CAD build for the part. Positions are in the model's coordinates, mm. A direction names the side the tool comes from. Coordinates: 2 decimals unless noted, no trailing zeros. Order: outer loops, then holes, each group sorted by start corner. A loop starts at its lowest first (then second) coordinate and runs counter-clockwise, first axis right, second up. Notation, with made-up numbers: (61, -10) -> (89, -10) arc R11 cw to (89, -4) -> close; hole circle Ø9 at (26, 69.25). An arc over 180 degrees is marked (long way). Use one line per item in the form item = value. Start each with the question number.
Autodesk Inventor part; units mm, degrees
ref_plane "YZ Plane" through (0, 0, 0) normal (1, 0, 0) x (0, 1, 0)
ref_plane "XZ Plane" through (0, 0, 0) normal (0, 1, 0) x (-1, 0, 0)
ref_plane "XY Plane" through (0, 0, 0) normal (0, 0, 1) x (1, 0, 0)
sketch "Sketch1" plane through (0, 0, 0) normal (0, 1, 0) x (-1, 0, 0)
  line L0 (15.875, -28.575) -> (-15.875, -28.575)
  line L1 (-15.875, -28.575) -> (-15.875, 28.575)
  line L2 (-15.875, 28.575) -> (15.875, 28.575)
  line L3 (15.875, 28.575) -> (15.875, -28.575)
  line L4 (15.875, -28.575) -> (-15.875, 28.575) construction
  line L5 (-15.875, -28.575) -> (15.875, 28.575) construction
  point P0 (0, 0)
  dimension "d0" = 31.75
  dimension "d1" = 57.15
extrude "Extrusion1" add sketch "Sketch1" along normal blind 9.525
sketch "Sketch2" plane through (0, 9.525, 0) normal (0, 1, 0) x (1, 0, 0)
  line L0 (15.875, -28.575) -> (15.875, 28.575)
  line L1 (-15.875, -28.575) -> (15.875, -28.575)
  line L2 (15.875, 28.575) -> (9.525, 28.575)
  line L3 (9.525, 28.575) -> (9.525, -28.575)
  line L4 (9.525, -28.575) -> (15.875, -28.575)
  line L5 (15.875, -28.575) -> (15.875, 28.575)
  point P0 (0, 0)
  dimension "d4" = 6.35
extrude "Extrusion2" add sketch "Sketch2" along normal blind 12.7
sketch "Sketch3" plane through (0, 0, 0) normal (0, -1, 0) x (1, 0, 0)
  line L0 (-15.875, 28.575) -> (9.525, 28.575)
  point P0 (0, 0)
  point P1 (4.699, -3.175)
  dimension "d14" = 4.826
  dimension "d15" = 31.75
hole "Hole1" at (4.699, 0, -3.175) direction (0, 1, 0) diameter 4.2 end through all counterbore diameter 7.62 counterbore depth 5.08
sketch "Sketch5" plane through (0, 9.525, 0) normal (0, 1, 0) x (1, 0, 0)
  line L0 (9.525, 28.575) -> (-15.875, 28.575)
  circle A0 centre (4.699, 3.175) radius 3.81
  line L1 (-15.875, -28.575) -> (9.525, -28.575)
  point P0 (0, 0)
  point P1 (-8.001, 3.175)
  dimension "d33" = 12.7
  dimension "d40" = 31.75
hole "Hole3" at (-8.001, 9.525, -3.175) direction (0, -1, 0) diameter 4.699 end through all counterbore diameter 7.62 counterbore depth 4.445
sketch "Sketch6" plane through (0, 0, 0) normal (0, -1, 0) x (1, 0, 0)
  circle A0 centre (-8.001, -8.179) radius 1.0125
  circle A1 centre (-8.001, 1.829) radius 1.0125
  circle A2 centre (-8.001, -3.175) radius 2.3495
  point P0 (0, 0)
  dimension "d34" = 2.025
  dimension "d35" = 2.025
  dimension "d36" = 5.004
  dimension "d37" = 5.004
extrude "Extrusion3" cut sketch "Sketch6" against normal blind 4.826 contours A0 | A1
properties part number "Mount for Slit VA100CP"
1) Cut at B-B on z = -4. Give the cut face in (x, y) (3 decimals).
2) Cut at C-C on z = -19. Give the cut face in (x, y) (3 decimals), then the cut area to 3 significant figures.
3) Cut at A-A on y = 3.75. Give the cut face in (x, z) (1 decimal).
4) Drop flat-ended pins along their axis: P1, Ø4, axis at x = -8.001, z = -3.175, coming from the +Y side; P2, Ø3, axis at x = 6, z = -1, coming from the +Y side (3 decimals); P3, Ø5.5, axis at x = 4.699, z = -3.175, coming from the -Y side; P4, Ø1.2, axis at x = -8.001, z = -8.179, coming from the -Y side. Give the stop position or say it passes through.
5) Cut at D-D on x = 2. Give the cut face in (y, z) (3 decimals).
6) Two-plate mould, pull along Z, no slides. Class faces 1 (the face through (-3, 9.525, 0)), 2 (the face through (4, 6, 28.575)), 3 (the face through (-9.013, 2.379, -8.134)): released by +Z, released by -Z, zero draft, split by the parting line, or undercut.
7) Probe L1, parallel to X at y = 2.5, z = -5 (3 decimals); L2, parallel to X at y = 11.75, z = -9.5 (3 decimals); L3, parallel to Y at x = -2, z = 15.5 (3 decimals). List the from-to ranges inside material, lowest first.
8) 3-axis set-ups, long thin cutter, end or side, ignore diameter. For faces 4 (the face through (-4.62, 7.27, -1.42)), 5 (the face through (7.017, 2.576, -0.152)), 6 (the face through (9.525, 16, 0)), 7 (the face through (-15.875, 5, 0)): which of +Z, -Z, +X, -X, +Y, -Y reach the whole face in a straight line?
Values follow:
q1.outline = (-15.875, 0) -> (-10.201, 0) -> (-10.201, 5.08) -> (-11.721, 5.08) -> (-11.721, 9.525) -> (-15.875, 9.525) -> close; (-5.801, 0) -> (0.979, 0) -> (0.979, 5.08) -> (2.768, 5.08) -> (2.768, 9.525) -> (-4.281, 9.525) -> (-4.281, 5.08) -> (-5.801, 5.08) -> close; (6.63, 5.08) -> (8.419, 5.08) -> (8.419, 0) -> (15.875, 0) -> (15.875, 22.225) -> (9.525, 22.225) -> (9.525, 9.525) -> (6.63, 9.525) -> close
q2.outline = (-15.875, 0) -> (15.875, 0) -> (15.875, 22.225) -> (9.525, 22.225) -> (9.525, 9.525) -> (-15.875, 9.525) -> close
q2.area = 383 mm^2
q3.outline = (-15.9, -28.6) -> (15.9, -28.6) -> (15.9, 28.6) -> (-15.9, 28.6) -> close; hole circle Ø4.7 at (-8, -3.2); hole circle Ø2 at (-8, -8.2); hole circle Ø2 at (-8, 1.8); hole circle Ø7.6 at (4.7, -3.2)
q4.P1 = through
q4.P2 = 9.525
q4.P3 = 5.08
q4.P4 = 4.83
q5.outline = (0, -28.575) -> (9.525, -28.575) -> (9.525, 28.575) -> (0, 28.575) -> (0, -0.486) -> (5.08, -0.486) -> (5.08, -5.864) -> (0, -5.864) -> close
q6.face_1 = zero draft
q6.face_2 = released by +Z
q6.face_3 = undercut
q7.L1 = -15.875 to -9.481, -6.521 to 1.355, 8.043 to 15.875
q7.L2 = 9.525 to 15.875
q7.L3 = 0 to 9.525
q8.face_4 = +Y
q8.face_5 = -Y
q8.face_6 = +Z, -Z, -X, +Y
q8.face_7 = +Z, -Z, -X, +Y, -Y
